Verification items for the finished model (mm, model axes). A direction names the side the tool comes from. Give positions to 0.01 mm unless a question says otherwise; leave off trailing zeros. Write each loop counter-clockwise with the first axis right and the second up, starting at its lowest first coordinate (ties: lowest second). Pieces come first, ordered by that corner, then holes. Notation, with made-up numbers: (-12, -17.5) -> (23, -17.5) arc R18 ccw to (23, -3.5) -> close; hole circle Ø6 at (68, -31). An arc over 180 degrees is marked (long way). Write item = value, one per line.
from build123d import *

# Parameters (mm, degrees)
PAD330_DEPTH         = 5
POCKET338_DEPTH      = 3
POCKET338_DEPTH_BACK = 3
SKETCH686_W          = 10
SKETCH686_H          = 2
POCKET342_DEPTH      = 5
POCKET342_DEPTH_BACK = 2
SKETCH674_W          = 10
SKETCH674_H          = 2
POCKET337_DEPTH      = 5
POCKET337_DEPTH_BACK = 2
POCKET337_FACE20_W   = 6
POCKET337_FACE20_H   = 5
POCKET344_DEPTH      = 5
POCKET344_FACE26_W   = 6
POCKET344_FACE26_H   = 5
POCKET349_DEPTH      = 5
PAD331_DEPTH         = 2
POCKET343_DEPTH      = 2
POCKET343_FACE66_W   = 6
POCKET343_FACE66_H   = 2.071068
POCKET352_DEPTH      = 5
POCKET352_FACE38_W   = 6
POCKET352_FACE38_H   = 2.071068
POCKET345_DEPTH      = 5


with BuildPart() as part:
    # Sketch675 → Pad330 (new body)
    with BuildSketch(Plane.XY):
        with BuildLine():
            Line((-10, -28.75), (10, -28.75))
            Line((10, -28.75), (10, 7.5))
            ThreePointArc((10, 7.5), (7.803301, 12.803301), (2.5, 15))
            Line((2.5, 15), (-2.5, 15))
            ThreePointArc((-2.5, 15), (-7.803301, 12.803301), (-10, 7.5))
            Line((-10, 7.5), (-10, -28.75))
        make_face()
    extrude(amount=PAD330_DEPTH)

    # Sketch666 → Pocket338 (cut, two sides)
    with BuildSketch(Plane.XZ) as pocket338_sk:
        Polygon((-10, 0), (-10, 5), (-8.585786, 6.414214), (-2.171573, 0), (-5, 0), align=None)
        Polygon((10, 0), (10, 5), (8.585786, 6.414214), (2.171573, 0), (5, 0), align=None)
    extrude(amount=-POCKET338_DEPTH, mode=Mode.SUBTRACT)
    extrude(pocket338_sk.sketch, amount=POCKET338_DEPTH_BACK, mode=Mode.SUBTRACT)

    # Sketch686 (on DatumPlane) → Pocket342 (cut, two sides)
    with BuildSketch(Plane(origin=(-7.171573, 3, 5), x_dir=(0, -1, 0), z_dir=(-0.707107, 0, 0.707107))) as pocket342_sk:
        with Locations((3, -1)):
            Rectangle(SKETCH686_W, SKETCH686_H)
    extrude(amount=-POCKET342_DEPTH, mode=Mode.SUBTRACT)
    extrude(pocket342_sk.sketch, amount=POCKET342_DEPTH_BACK, mode=Mode.SUBTRACT)

    # Sketch674 (on DatumPlane) → Pocket337 (cut, two sides)
    with BuildSketch(Plane(origin=(7.171573, 3, 5), x_dir=(0, 1, 0), z_dir=(0.707107, 0, 0.707107))) as pocket337_sk:
        with Locations((-3, -1)):
            Rectangle(SKETCH674_W, SKETCH674_H)
    extrude(amount=-POCKET337_DEPTH, mode=Mode.SUBTRACT)
    extrude(pocket337_sk.sketch, amount=POCKET337_DEPTH_BACK, mode=Mode.SUBTRACT)

    # Pocket337 Face20 → Pocket344 (cut)
    with BuildSketch(Plane(origin=(-5.403806, 0, 3.232233), x_dir=(0, 1, 0), z_dir=(-0.707107, 0, -0.707107))):
        Rectangle(POCKET337_FACE20_W, POCKET337_FACE20_H)
    extrude(amount=-POCKET344_DEPTH, mode=Mode.SUBTRACT)

    # Pocket344 Face26 → Pocket349 (cut)
    with BuildSketch(Plane(origin=(5.403806, 0, 3.232233), x_dir=(0, -1, 0), z_dir=(0.707107, 0, -0.707107))):
        Rectangle(POCKET344_FACE26_W, POCKET344_FACE26_H)
    extrude(amount=-POCKET349_DEPTH, mode=Mode.SUBTRACT)

    # Pocket349 Face4 → Pad331 (add)
    with BuildSketch(Plane(origin=(0, -8.372552, 0), x_dir=(0, -1, 0), z_dir=(0, 0, -1))):
        with BuildLine():
            Line((20.377448, 10), (-5.372552, 10))
            Line((-5.372552, 10), (-5.372552, 5))
            Line((-5.372552, 5), (-5.372552, 2.171573))
            Line((-5.372552, 2.171573), (-11.372552, 2.171573))
            Line((-11.372552, 2.171573), (-11.372552, 5))
            Line((-11.372552, 5), (-11.372552, 10))
            Line((-11.372552, 10), (-15.872552, 10))
            ThreePointArc((-15.872552, 10), (-21.175853, 7.803301), (-23.372552, 2.5))
            Line((-23.372552, 2.5), (-23.372552, -2.5))
            ThreePointArc((-23.372552, -2.5), (-21.175853, -7.803301), (-15.872552, -10))
            Line((-15.872552, -10), (-11.372552, -10))
            Line((-11.372552, -10), (-11.372552, -5))
            Line((-11.372552, -5), (-11.372552, -2.171573))
            Line((-11.372552, -2.171573), (-5.372552, -2.171573))
            Line((-5.372552, -2.171573), (-5.372552, -5))
            Line((-5.372552, -5), (-5.372552, -10))
            Line((-5.372552, -10), (20.377448, -10))
            Line((20.377448, -10), (20.377448, 10))
        make_face()
    extrude(amount=PAD331_DEPTH)

    # Pad331 Face5 → Pocket343 (cut)
    with BuildSketch(Plane(origin=(0, -8.9329, 5), x_dir=(0, 1, 0), z_dir=(0, 0, 1))):
        with BuildLine():
            Line((11.9329, 0.100505), (5.9329, 0.100505))
            Line((5.9329, 0.100505), (5.9329, 7.171573))
            Line((5.9329, 7.171573), (3.9329, 7.171573))
            Line((3.9329, 7.171573), (3.9329, 10))
            Line((3.9329, 10), (-19.8171, 10))
            Line((-19.8171, 10), (-19.8171, -10))
            Line((-19.8171, -10), (3.9329, -10))
            Line((3.9329, -10), (3.9329, -7.171573))
            Line((3.9329, -7.171573), (5.9329, -7.171573))
            Line((5.9329, -7.171573), (5.9329, -0.100505))
            Line((5.9329, -0.100505), (11.9329, -0.100505))
            Line((11.9329, -0.100505), (11.9329, -7.171573))
            Line((11.9329, -7.171573), (13.9329, -7.171573))
            Line((13.9329, -7.171573), (13.9329, -10))
            Line((13.9329, -10), (16.4329, -10))
            ThreePointArc((16.4329, -10), (21.736201, -7.803301), (23.9329, -2.5))
            Line((23.9329, -2.5), (23.9329, 2.5))
            ThreePointArc((23.9329, 2.5), (21.736201, 7.803301), (16.4329, 10))
            Line((16.4329, 10), (13.9329, 10))
            Line((13.9329, 10), (13.9329, 7.171573))
            Line((13.9329, 7.171573), (11.9329, 7.171573))
            Line((11.9329, 7.171573), (11.9329, 0.100505))
        make_face()
    extrude(amount=-POCKET343_DEPTH, mode=Mode.SUBTRACT)

    # Pocket343 Face66 → Pocket352 (cut)
    with BuildSketch(Plane(origin=(-2.903806, 0, 0.732233), x_dir=(0, 1, 0), z_dir=(-0.707107, 0, -0.707107))):
        Rectangle(POCKET343_FACE66_W, POCKET343_FACE66_H)
    extrude(amount=-POCKET352_DEPTH, mode=Mode.SUBTRACT)

    # Pocket352 Face38 → Pocket345 (cut)
    with BuildSketch(Plane(origin=(2.903806, 0, 0.732233), x_dir=(0, -1, 0), z_dir=(0.707107, 0, -0.707107))):
        Rectangle(POCKET352_FACE38_W, POCKET352_FACE38_H)
    extrude(amount=-POCKET345_DEPTH, mode=Mode.SUBTRACT)


with BuildPart() as part_1:
    # Body211 placement: moved
    add(part.part.moved(Location((0, 103.75, 2))))


solid = part_1.part
Item 1: Sectioned sample at A-A on z = 5.5. Record the cut outline in (x, y), then the cut area to 3 significant figures.
Response values:
outline = (-10, 98.75) -> (-8.5, 98.75) -> (-8.5, 100.75) -> (-10, 100.75) -> close; (-10, 106.75) -> (-8.5, 106.75) -> (-8.5, 108.75) -> (-10, 108.75) -> close; (8.5, 98.75) -> (10, 98.75) -> (10, 100.75) -> (8.5, 100.75) -> close; (8.5, 106.75) -> (10, 106.75) -> (10, 108.75) -> (8.5, 108.75) -> close
area = 12.0 mm^2
Item 2: Go/stop test with flat-tipped pins: P1, Ø6, axis at x = 3, y = 86, coming from the +Z side; P2, Ø1.6, axis at y = 104.5, z = 0.5, coming from the +X side; P3, Ø1.5, axis at x = -5, z = 4, coming from the +Y side; P4, Ø1, axis at x = 8.5, z = 6.5, coming from the +Y side. Record where each tip stops, or that it passes through.
Response values:
P1 = 5
P2 = 2.17
P3 = 118.54
P4 = through
Item 3: Set-up check for faces 4 (the flat face through (-1.1, 103.71, 3.07)), 5 (the flat face through (-5, 108.75, 4)), 6 (the flat face through (0, 113, 5)), 7 (the flat face through (-9.4, 98.75, 5.6)): record each of +Z, -Z, +X, -X, +Y, -Y from which the full face is reachable in a straight line by a thin tool's end or side.
Response values:
face_4 = +Z, -X
face_5 = none
face_6 = +Z, +Y
face_7 = +Z, +X, -X, -Y
Item 4: Mould release check, pull along X, two halves, no side actions. Record for faces 1 (the flat face through (10, 88, 3)), 2 (the flat face through (4.3, 99.7, 2.8)), 3 (the flat face through (-10, 88, 3)): +X half, -X half, draft (parallel to the pull), parting line (faces both ways), or undercut.
Response values:
face_1 = +X half
face_2 = undercut
face_3 = -X half
Item 5: Sectioned sample at B-B on x = 8.5. Record the cut outline in (y, z), then the cut area to 3 significant figures.
Response values:
outline = (75, 0) -> (100.75, 0) -> (100.75, 5.5) -> (98.75, 5.5) -> (98.75, 5) -> (75, 5) -> close; (106.75, 0) -> (115.75, 0) -> (115.75, 5) -> (108.75, 5) -> (108.75, 5.5) -> (106.75, 5.5) -> close
area = 176 mm^2
Item 6: Sectioned sample at C-C on z = 1.5. Record the cut outline in (x, y).
Response values:
outline = (-10, 75) -> (10, 75) -> (10, 100.75) -> (2.17, 100.75) -> (2.17, 106.75) -> (10, 106.75) -> (10, 111.25) arc R7.5 ccw to (2.5, 118.75) -> (-2.5, 118.75) arc R7.5 ccw to (-10, 111.25) -> (-10, 106.75) -> (-2.17, 106.75) -> (-2.17, 100.75) -> (-10, 100.75) -> close
Item 7: Sectioned sample at D-D on x = 1.25. Record the cut outline in (y, z).
Response values:
outline = (75, 0) -> (118.75, 0) -> (118.75, 5) -> (106.75, 5) -> (106.75, 2.92) -> (100.75, 2.92) -> (100.75, 5) -> (75, 5) -> close
Item 8: Material ranges on line 1 (Y direction, x = 0, z = 4.25); line 2 (X direction, y = 100.5, z = 4.25); line 3 (Z direction, x = 3, y = 82.5), recorded low to high.
Response values:
line_1 = 75 to 100.75, 106.75 to 118.75
line_2 = -10 to -7.25, -4.42 to 4.42, 7.25 to 10
line_3 = 0 to 5
